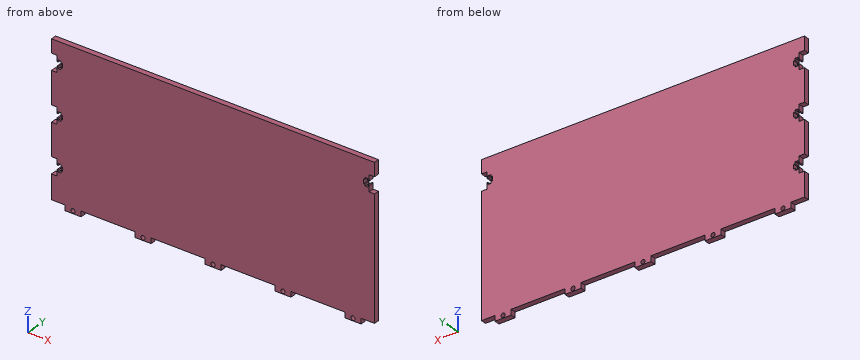
from build123d import *

# Parameters (mm, degrees)
SKETCH1_W                    = 381
SKETCH1_H                    = 177.8
BOSS_EXTRUDE1_DEPTH          = 6.35
SKETCH2_W                    = 19.05
SKETCH2_H                    = 6.35
BOSS_EXTRUDE2_DEPTH          = 6.35
F_10_0_1935_DIAMETER_HOLE1_D = 4.9149
LPATTERN1_COUNT              = 5
LPATTERN1_PITCH              = 82.55
CUT_EXTRUDE2_DEPTH           = 424.216900655
LPATTERN4_COUNT              = 3
LPATTERN4_PITCH              = 57.15


with BuildPart() as part:
    # Sketch1 → Boss-Extrude1 (new body)
    with BuildSketch(Plane(origin=(0, 0, 0), x_dir=(1, 0, 0), z_dir=(0, 1, 0))):
        with Locations((190.5, 88.9)):
            Rectangle(SKETCH1_W, SKETCH1_H)
    extrude(amount=BOSS_EXTRUDE1_DEPTH)

    # Sketch2 → Boss-Extrude2 (add)
    with BuildSketch(Plane(origin=(0, 6.35, 0), x_dir=(1, 0, 0), z_dir=(0, 1, 0))):
        with Locations((25.4, 180.975)):
            Rectangle(SKETCH2_W, SKETCH2_H)
    boss_extrude2 = extrude(amount=-BOSS_EXTRUDE2_DEPTH)

    # #10 (0.1935) Diameter Hole1 (through all)
    with Locations(Plane(origin=(0, 6.35, 0), x_dir=(1, 0, 0), z_dir=(0, 1, 0))):
        with Locations((25.4, 180.975)):
            f_10_0_1935_diameter_hole1 = Hole(F_10_0_1935_DIAMETER_HOLE1_D / 2)

    # LPattern1: Boss-Extrude2, #10 (0.1935) Diameter Hole1 ×5
    with Locations(*[(i * LPATTERN1_PITCH, 0, 0) for i in range(1, LPATTERN1_COUNT)]):
        add(boss_extrude2)
        add(f_10_0_1935_diameter_hole1, mode=Mode.SUBTRACT)

    # Sketch7 → Cut-Extrude2 (cut, through all)
    with BuildSketch(Plane(origin=(0, 6.35, 0), x_dir=(1, 0, 0), z_dir=(0, 1, 0))):
        Polygon((0, 34.925), (0, 15.875), (6.35, 15.875), (6.35, 22.86), (7.874, 22.86), (7.874, 20.574), (11.176, 20.574), (11.176, 22.86), (12.7, 22.86), (12.7, 27.94), (11.176, 27.94), (11.176, 30.226), (7.874, 30.226), (7.874, 27.94), (6.35, 27.94), (6.35, 34.925), align=None)
    cut_extrude2 = extrude(amount=-CUT_EXTRUDE2_DEPTH, mode=Mode.SUBTRACT)

    # Mirror2: Cut-Extrude2 across plane
    add(cut_extrude2.mirror(Plane.ZY.offset(-190.5)), mode=Mode.SUBTRACT)

    # LPattern4: Cut-Extrude2 ×3
    with Locations(*[(0, 0, -i * LPATTERN4_PITCH) for i in range(1, LPATTERN4_COUNT)]):
        add(cut_extrude2, mode=Mode.SUBTRACT)


solid = part.part
Work out the finished part from the listing and answer in its coordinate system (mm). Round coordinates to 2 decimals unless told otherwise and drop trailing zeros. Loops run counter-clockwise (first coordinate to the right, second up) from the corner with the lowest first, then second, coordinate; pieces in that order, holes last. Notation, with made-up numbers: M 20.25,11 L 68.25,11 A22 cw 68.25,29 Z; hole C 57,37 d5. An arc over 180 degrees is marked long. One line per question, with ' | ' between items. Start each with the question number.
(1) Flat-ended cylindrical pins translate along their axes: pin 1 Ø4 at (x, z) = (355.6, -180.975) entering from -Y; pin 2 Ø1.2 at (x, y) = (374, 3.5) entering from -Z; pin 3 Ø1.8 at (y, z) = (4.5, -21.5) entering from -X; pin 4 Ø2.5 at (y, z) = (4.5, -21.5) entering from +X. Find the tip coordinate at first contact, or state that the pin passes through.
(2) Find the intervals of material crossed by line 1 (Z direction, x = 273.05, y = 3.75); line 2 (X direction, y = 2.75, z = -137.5); line 3 (Z direction, x = 263, y = 2.5), in increasing order.
(3) A cutting plane is placed at A-A on x = 247. Write down the section's boundary in (y, z).
(4) A cutting plane is placed at B-B on y = 1.25. Give the number of separate pieces and of enclosed holes in the cut face, plus the area to 3 significant figures.
Geometry check:
1) pin 1: passes through | pin 2: stops at z = -177.8 | pin 3: stops at x = 6.35 | pin 4: stops at x = 374.65
2) line 1: z = -184.15 to -183.43, -178.52 to 0 | line 2: x = 12.7 to 381 | line 3: z = -177.8 to 0
3) outline: M 0,-177.8 L 6.35,-177.8 L 6.35,0 L 0,0 Z
4) separate pieces: 1 | enclosed holes: 5 | area: 67,600 mm²
